The listing builds one solid part. Answer for the finished solid, in the listing's coordinates (mm). A direction names the side the tool comes from. Coordinates: 2 decimals unless noted, no trailing zeros. Order: outer loops, then holes, each group sorted by start corner. A loop starts at its lowest first (then second) coordinate and runs counter-clockwise, first axis right, second up. Notation, with made-up numbers: (23.25, 36) -> (42.25, 36) arc R28 cw to (42.25, 75) -> close; hole circle Ø9 at (-28, 61.25). An arc over 180 degrees is marked (long way). Put each result on its own line as item: value. Start each with the question number.
Autodesk Inventor part; units mm, degrees
ref_plane "YZ Plane" through (0, 0, 0) normal (1, 0, 0) x (0, 1, 0)
ref_plane "XZ Plane" through (0, 0, 0) normal (0, 1, 0) x (-1, 0, 0)
ref_plane "XY Plane" through (0, 0, 0) normal (0, 0, 1) x (1, 0, 0)
sketch "Sketch1" plane through (0, 0, 0) normal (0, 0, 1) x (1, 0, 0)
  line L0 (-51.5087, 0.9312) -> (-0.7087, 0.9312)
  line L1 (-0.7087, 0.9312) -> (-0.7087, 11.0912)
  line L2 (-0.7087, 11.0912) -> (-51.5087, 11.0912)
  line L3 (-51.5087, 11.0912) -> (-51.5087, 0.9312)
  dimension "d1" = 10.16
  dimension "d2" = 50.8
extrude "Extrusion1" add sketch "Sketch1" along normal blind 50.8
sketch "Sketch2" plane through (0, 0, 0) normal (0, 0, -1) x (-1, 0, 0)
  arc A0 (43.6087, 20.9733) -> (43.6087, 27.9733) centre (43.6087, 24.4733) ccw
  line L0 (8.6087, 27.9733) -> (12.5532, 27.9733)
  line L1 (8.6087, 27.9733) -> (12.5532, 27.9733)
  line L2 (8.6087, 20.9733) -> (12.5532, 20.9733)
  line L3 (8.6087, 20.9733) -> (12.5532, 20.9733)
  arc A1 (9.0398, 27.9733) -> (9.0398, 20.9733) centre (8.6512, 24.4733) ccw
  line L4 (43.6087, 27.9733) -> (39.6641, 27.9733)
  line L5 (39.6641, 27.9733) -> (43.6087, 27.9733)
  line L6 (43.6087, 20.9733) -> (39.6641, 20.9733)
  line L7 (39.6641, 20.9733) -> (43.6087, 20.9733)
  arc A2 (18.8087, 11.9789) -> (18.362, 12.8118) centre (17.8087, 11.9789) ccw
  line L8 (18.8087, 8.6771) -> (18.8087, 11.5509)
  line L9 (18.8087, 11.9789) -> (18.8087, 8.6771)
  line L10 (18.8087, 8.6771) -> (18.8087, 7.6771)
  arc A3 (18.8087, 8.6771) -> (19.8087, 7.6771) centre (19.8087, 8.6771) ccw
  line L11 (18.8087, 7.6771) -> (33.4087, 7.6771)
  line L12 (33.4087, 11.9789) -> (33.4087, 11.5509)
  line L13 (33.4087, 7.6771) -> (33.4087, 11.9789)
  arc A4 (33.8554, 12.8118) -> (33.4087, 11.9789) centre (34.4087, 11.9789) ccw
  arc A5 (33.4087, 11.9789) -> (33.4087, 11.9789) centre (34.4087, 11.9789) ccw
  arc A6 (18.8087, 11.9789) -> (18.362, 12.8118) centre (17.8087, 11.9789) ccw
  arc A7 (12.5532, 20.9733) -> (18.362, 12.8118) centre (26.1087, 24.4733) ccw
  arc A8 (33.8554, 12.8118) -> (39.6641, 20.9733) centre (26.1087, 24.4733) ccw
  arc A9 (39.6641, 27.9733) -> (12.5532, 27.9733) centre (26.1087, 24.4733) ccw
  line L14 (0.7087, 11.0912) -> (51.5087, 11.0912)
  circle A10 centre (26.1087, 24.4733) radius 14
  line L15 (0.7087, 0.9312) -> (0.7087, 11.0912)
  line L16 (0.7087, 11.0912) -> (51.5087, 11.0912)
  line L17 (51.5087, 11.0912) -> (51.5087, 61.8912)
  line L18 (51.5087, 61.8912) -> (0.7087, 61.8912)
  line L19 (0.7087, 61.8912) -> (0.7087, 11.0912)
  line L20 (11.3767, 28.2833) -> (11.3767, 11.0912)
  line L21 (11.3767, 28.2833) -> (11.3767, 44.1112)
  line L22 (11.3767, 44.1112) -> (40.8407, 44.1112)
  line L23 (40.8407, 44.1112) -> (40.8407, 11.0912)
  point P0 (0, 0)
  point P1 (26.1087, 11.0912)
  dimension "d6" = 0
  dimension "d7" = 50.8
  dimension "d9" = 14.732
  dimension "d10" = 14.732
  dimension "d11" = 33.02
extrude "Extrusion2" add sketch "Sketch2" against normal blind 6.35 contours L6 L23 L4 A0 | A0 L4 L23 L22 L21 L20 L0 A1 L2 L14 L19 L18 L17 L6 | L20 L2 A1 L0
sketch "Sketch3" plane through (0, 0, 0) normal (0, 0, -1) x (-1, 0, 0)
  arc A0 (43.6087, 24.541) -> (43.6087, 31.541) centre (43.6087, 28.041) ccw
  line L0 (8.6087, 31.541) -> (12.5532, 31.541)
  line L1 (8.6087, 31.541) -> (12.5532, 31.541)
  line L2 (8.6087, 24.541) -> (12.5532, 24.541)
  line L3 (8.6087, 24.541) -> (12.5532, 24.541)
  arc A1 (9.0398, 31.541) -> (9.0398, 24.541) centre (8.6512, 28.041) ccw
  line L4 (43.6087, 31.541) -> (39.6641, 31.541)
  line L5 (39.6641, 31.541) -> (43.6087, 31.541)
  line L6 (43.6087, 24.541) -> (39.6641, 24.541)
  line L7 (39.6641, 24.541) -> (43.6087, 24.541)
  arc A2 (18.8087, 15.5466) -> (18.362, 16.3795) centre (17.8087, 15.5466) ccw
  line L8 (18.8087, 12.2448) -> (18.8087, 15.1185)
  line L9 (18.8087, 15.5466) -> (18.8087, 12.2448)
  line L10 (18.8087, 12.2448) -> (18.8087, 11.2448)
  arc A3 (18.8087, 12.2448) -> (19.8087, 11.2448) centre (19.8087, 12.2448) ccw
  line L11 (18.8087, 11.2448) -> (33.4087, 11.2448)
  line L12 (33.4087, 15.5466) -> (33.4087, 15.1185)
  line L13 (33.4087, 11.2448) -> (33.4087, 15.5466)
  arc A4 (33.8554, 16.3795) -> (33.4087, 15.5466) centre (34.4087, 15.5466) ccw
  arc A5 (33.4087, 15.5466) -> (33.4087, 15.5466) centre (34.4087, 15.5466) ccw
  arc A6 (18.8087, 15.5466) -> (18.362, 16.3795) centre (17.8087, 15.5466) ccw
  arc A7 (12.5532, 24.541) -> (18.362, 16.3795) centre (26.1087, 28.041) ccw
  arc A8 (33.8554, 16.3795) -> (39.6641, 24.541) centre (26.1087, 28.041) ccw
  arc A9 (39.6641, 31.541) -> (12.5532, 31.541) centre (26.1087, 28.041) ccw
  line L14 (11.3767, 11.0912) -> (40.8407, 11.0912)
  circle A10 centre (26.1087, 28.041) radius 25.7175
  circle A11 centre (26.1087, 61.7236) radius 7.62
  line L15 (0.7087, 61.8912) -> (51.5087, 61.8912)
  line L16 (0.7087, 0.9312) -> (0.7087, 61.8912)
  line L17 (0.7087, 61.8912) -> (51.5087, 61.8912)
  line L18 (51.5087, 61.8912) -> (51.5087, 76.3692)
  line L19 (51.5087, 76.3692) -> (0.7087, 76.3692)
  line L20 (0.7087, 76.3692) -> (0.7087, 61.8912)
  point P0 (0, 0)
  point P1 (26.1087, 11.0912)
  point P2 (26.1087, 61.8912)
  dimension "d15" = 0
  dimension "d16" = 51.435
  dimension "d17" = 15.24
  dimension "d18" = 0
  dimension "d19" = 14.478
extrude "Extrusion3" add sketch "Sketch3" against normal blind 6.35 contours L20 L19 L18 L15 A11 | A11 L15 picked at (24.5986, 64.5356)
sketch "Sketch5" plane through (0, 0, 0) normal (0, 0, -1) x (-1, 0, 0)
  line L0 (0.7087, 11.0912) -> (51.5087, 11.0912)
  line L1 (26.1087, 11.0912) -> (26.1087, 35.6872)
  line L2 (26.1087, 35.6872) -> (26.1087, 61.4047)
  circle A0 centre (26.1087, 72.7077) radius 7.62
  circle A1 centre (26.1087, 72.7077) radius 1.905
  line L3 (0.7087, 76.3692) -> (51.5087, 76.3692)
  point P0 (0, 0)
  dimension "d26" = 24.596
  dimension "d27" = 25.7175
  dimension "d28" = 15.24
  dimension "d29" = 11.303
  dimension "d30" = 3.81
extrude "Extrusion5" cut sketch "Sketch5" against normal up to next contours A1
sketch "Sketch6" plane through (0, 0, 0) normal (0, 0, -1) x (-1, 0, 0)
  line L0 (0.7087, 76.3692) -> (51.5087, 76.3692)
  line L1 (0.7087, 76.3692) -> (51.5087, 76.3692)
  line L2 (51.5087, 76.3692) -> (51.5087, 87.1857)
  line L3 (51.5087, 87.1857) -> (0.7087, 87.1857)
  line L4 (0.7087, 87.1857) -> (0.7087, 76.3692)
  circle A0 centre (26.1087, 72.7077) radius 1.905
  point P0 (0, 0)
  dimension "d33" = 14.478
extrude "Extrusion6" add sketch "Sketch6" against normal blind 6.35 contours L4 L3 L2 L0
sketch "Sketch8" plane through (-51.5087, 11.0912, 50.8) normal (0, 1, 0) x (1, 0, 0)
  circle A0 centre (40.64, 10.16) radius 2.3813
  circle A1 centre (10.16, 10.16) radius 2.3813
  line L0 (50.8, 0) -> (0, 0)
  line L1 (50.8, 50.8) -> (50.8, 0)
  line L2 (0, 44.45) -> (0, 0)
  point P0 (51.5087, 50.8)
  dimension "d36" = 4.7625
  dimension "d37" = 4.7625
  dimension "d38" = 10.16
  dimension "d39" = 10.16
  dimension "d40" = 10.16
  dimension "d41" = 10.16
extrude "Extrusion7" cut sketch "Sketch8" against normal up to next
sketch "Sketch9" plane through (0, 0, 0) normal (0, 0, -1) x (-1, 0, 0)
  line L0 (11.3767, 11.0912) -> (40.8407, 11.0912)
  line L1 (26.1087, 11.0912) -> (26.1087, 0.9312)
  line L2 (51.5087, 0.9312) -> (0.7087, 0.9312)
  line L3 (22.9337, 11.0912) -> (29.2837, 11.0912)
  line L4 (29.2837, 11.0912) -> (29.2837, 0.9312)
  line L5 (29.2837, 0.9312) -> (22.9337, 0.9312)
  line L6 (22.9337, 0.9312) -> (22.9337, 11.0912)
  point P0 (0, 0)
  dimension "d45" = 6.35
  dimension "d46" = 3.175
extrude "Extrusion8" cut sketch "Sketch9" against normal blind 25.4
sketch "Sketch10" plane through (0, 0, 0) normal (0, 0, -1) x (-1, 0, 0)
  point P0 (0, 0)
properties part number "End Frame 2"
(1) A tool of negligible diameter and unlimited length cuts with its end or side. For faces 5 (the flat face through (-26, 58, 6.35)), 6 (the flat face through (-11.377, 27, 3)), 7 (the flat face through (-26, 6, 25.4)), from which of +Z, -Z, +X, -X, +Y, -Y can it reach the whole face along a straight path? Write none if from no direction.
(2) Each of these flat-tipped pins is pushed along its axis until it touches: P1, Ø1.5, axis at x = -15, z = 42, coming from the +Y side; P2, Ø3, axis at x = -26.11, y = 72.71, coming from the +Z side; P3, Ø8, axis at x = -31.5, y = 60, coming from the +Z side. Where does it stop, or does it pass through?
(3) The part is cut by section C-C on z = 40.64. Determine the outline of the cut face in (x, y), plus the area to 3 significant figures.
(4) The part is cut by section A-A on y = 18. Determine the outline of the cut face in (x, z), plus the area to 3 significant figures.
(5) For a pull along X with two mould halves and no side action, classify faces 1 (the flat face through (-26, 44.111, 3)), 2 (the cylindrical face through (-8.6, 6.08, 39.92)), 3 (the flat face through (-51.509, 25, 5)), 4 (the flat face through (-26, 45, 0)) as released by +X, released by -X, zero draft, split by the parting line, or undercut.
(6) The part is cut by section B-B on x = -15. Determine the outline of the cut face in (y, z), plus the area to 3 significant figures.
(7) The part is cut by section D-D on z = 4. Determine the outline of the cut face in (x, y) (3 decimals), plus the area to 3 significant figures.
(8) Find the intervals of material crossed by L1, parallel to X at y = 7.5, z = 40.64; L2, parallel to X at y = 4, z = 40; L3, parallel to Z at x = -21, y = 61.5, in increasing order.
Worked out:
1. face 5: +Z, +X, -X, +Y
1. face 6: +Z, -Z
1. face 7: -Z, +Y, -Y
2. P1: y = 11.09
2. P2: through
2. P3: z = 6.35
3. outline: (-51.51, 0.93) -> (-43.73, 0.93) -> (-43.73, 11.09) -> (-51.51, 11.09) -> close; (-38.97, 0.93) -> (-13.25, 0.93) -> (-13.25, 11.09) -> (-38.97, 11.09) -> close; (-8.49, 0.93) -> (-0.71, 0.93) -> (-0.71, 11.09) -> (-8.49, 11.09) -> close
3. area: 419 mm2
4. outline: (-51.51, 0) -> (-40.84, 0) -> (-40.84, 6.35) -> (-51.51, 6.35) -> close; (-11.38, 0) -> (-0.71, 0) -> (-0.71, 6.35) -> (-11.38, 6.35) -> close
4. area: 135 mm2
5. face 1: undercut
5. face 2: undercut
5. face 3: released by -X
5. face 4: zero draft
6. outline: (0.93, 0) -> (11.09, 0) -> (11.09, 50.8) -> (0.93, 50.8) -> close; (44.11, 0) -> (87.19, 0) -> (87.19, 6.35) -> (44.11, 6.35) -> close
6. area: 790 mm2
7. outline: (-51.509, 0.931) -> (-29.284, 0.931) -> (-29.284, 11.091) -> (-40.841, 11.091) -> (-40.841, 44.111) -> (-11.377, 44.111) -> (-11.377, 11.091) -> (-22.934, 11.091) -> (-22.934, 0.931) -> (-0.709, 0.931) -> (-0.709, 87.186) -> (-51.509, 87.186) -> close; hole circle Ø3.81 at (-26.109, 72.708)
7. area: 3,330 mm2
8. L1: -51.51 to -43.73, -38.97 to -13.25, -8.49 to -0.71
8. L2: -51.51 to -43.64, -39.06 to -13.16, -8.58 to -0.71
8. L3: 0 to 6.35
